Autodesk Fusion 360 part; units mm, degrees
sketch "Sketch1" plane through (0, 0, 0) normal (0, 0, 1) x (1, 0, 0)
  line L0 (25, -25) -> (-25, -25)
  line L1 (-25, -25) -> (-25, 25)
  line L2 (-25, 25) -> (25, 25)
  line L3 (25, 25) -> (25, -25)
  line L4 (25, -25) -> (-25, 25) construction
  line L5 (-25, -25) -> (25, 25) construction
  dimension "d1" = 50
  dimension "d2" = 50
extrude "Extrude1" add sketch "Sketch1" along normal blind 65
fillet "Fillet1" radius 2 4 edges at (-25, -25, 32.5) (25, -25, 32.5) (-25, 25, 32.5) (25, 25, 32.5)
shell "Shell1" thickness 1.6 removed faces 1 at (7.6667, -8.3333, 65)
sketch "Sketch2" plane through (0, 0, 65) normal (0, 0, 1) x (-1, 0, 0)
  arc A0 (-23, 23.4) -> (-23.4, 23) centre (-23, 23) ccw
  line L0 (-23, 23.4) -> (23, 23.4)
  arc A1 (23.4, 23) -> (23, 23.4) centre (23, 23) ccw
  line L1 (23.4, 23) -> (23.4, -23)
  arc A2 (23, -23.4) -> (23.4, -23) centre (23, -23) ccw
  line L2 (23, -23.4) -> (-23, -23.4)
  arc A3 (-23.4, -23) -> (-23, -23.4) centre (-23, -23) ccw
  line L3 (-23.4, -23) -> (-23.4, 23)
  arc A4 (-25, -23) -> (-23, -25) centre (-23, -23) ccw
  line L4 (-23, -25) -> (23, -25)
  arc A5 (23, -25) -> (25, -23) centre (23, -23) ccw
  line L5 (25, -23) -> (25, 23)
  arc A6 (25, 23) -> (23, 25) centre (23, 23) ccw
  line L6 (23, 25) -> (-23, 25)
  arc A7 (-23, 25) -> (-25, 23) centre (-23, 23) ccw
  line L7 (-25, 23) -> (-25, -23)
extrude "Extrude2" add sketch "Sketch2" against normal blind 1.6 contours A0 L0 A1 L1 A2 L2 A3 L3
Work out the finished part from the listing and answer in its coordinate system (mm). A direction names the side the tool comes from. Give positions to 0.01 mm unless a question says otherwise; leave off trailing zeros. Write each loop counter-clockwise with the first axis right and the second up, starting at its lowest first coordinate (ties: lowest second). Pieces come first, ordered by that corner, then holes. Notation, with made-up numbers: (40, 88) - (98, 88) arc R17 ccw to (98, 97) - close; hole circle Ø3 at (-20, 84.25). An arc over 180 degrees is marked (long way). Use one line per item in the form item = value.
1. A cutting plane is placed at B-B (z = 17). Write down the section's boundary in (x, y), and give its area (3 significant figures).
Filled in:
outline = (-25, -23) arc R2 ccw to (-23, -25) - (23, -25) arc R2 ccw to (25, -23) - (25, 23) arc R2 ccw to (23, 25) - (-23, 25) arc R2 ccw to (-25, 23) - close; hole (-23.4, -23) arc R0.4 ccw to (-23, -23.4) - (23, -23.4) arc R0.4 ccw to (23.4, -23) - (23.4, 23) arc R0.4 ccw to (23, 23.4) - (-23, 23.4) arc R0.4 ccw to (-23.4, 23) - close
area = 306 mm^2
2. A cutting plane is placed at A-A (y = -22). Write down the section's boundary in (x, z), and give its area (3 significant figures).
Filled in:
outline = (-25, 0) - (25, 0) - (25, 65) - (-25, 65) - close; hole (-23.4, 1.6) - (23.4, 1.6) - (23.4, 63.4) - (-23.4, 63.4) - close
area = 358 mm^2
3. This flat-tipped pin is pushed along its axis until it touches: pin 1 Ø14 at (x, y) = (8, 0.5) entering from -Z. Where does it stop, or does it pass through?
Filled in:
pin_1 = 0
4. Consider L1, parallel to Y at x = -1, z = 56; L2, parallel to Z at x = 18, y = 3. Determine where each line is inside the solid, lowest interval first.
Filled in:
L1 = -25 to -23.4, 23.4 to 25
L2 = 0 to 1.6, 63.4 to 65
5. For faces 1 (the face through (0, 23.4, 32)), 2 (the face through (24.4, -24.43, 32.96)), determine the directions among +Z, -Z, +X, -X, +Y, -Y from which every point of the face is accessible in a straight line to the end or side of a thin tool.
Filled in:
face_1 = none
face_2 = +Z, -Z, +X, -Y
6. Determine the mould class of faces 3 (the face through (0, -25, 32)), 4 (the face through (0, 0, 0)), 5 (the face through (0, 0, 1.6)) for opening direction Y: released by +Y, released by -Y, zero draft, split by the parting line, or undercut.
Filled in:
face_3 = released by -Y
face_4 = zero draft
face_5 = undercut
